Source: CAD feature listing. Evaluate the final solid. Frame: model axes, mm. A direction names the side the tool comes from. Give positions to 0.01 mm unless a question says otherwise; leave off trailing zeros. Loops run counter-clockwise (first coordinate to the right, second up) from the corner with the lowest first, then second, coordinate; pieces in that order, holes last. Notation, with made-up numbers: (-35.75, -3) - (-18.75, -3) arc R24 ccw to (-18.75, 22) - close; hole circle Ø10 at (79.25, 44.25). An arc over 180 degrees is marked (long way). Put each result on its own line as item: value.
```python
from build123d import *

# Parameters (mm, degrees)
BOSS_EXTRUDE1_DEPTH = 2.9972
FILLET1_R           = 1.27


with BuildPart() as part:
    # Sketch1 → Boss-Extrude1 (new body)
    with BuildSketch(Plane.XY):
        with BuildLine():
            Line((0, 0), (0, 15.24))
            Line((0, 15.24), (2.117246866, 15.24))
            ThreePointArc((2.117246866, 15.24), (6.0706, 8.001), (10.023953134, 15.24))
            Line((10.023953134, 15.24), (12.1412, 15.24))
            Line((12.1412, 15.24), (12.1412, 0))
            Line((12.1412, 0), (7.5692, 0))
            Line((7.5692, 0), (7.5692, 3.175))
            Line((7.5692, 3.175), (4.572, 3.175))
            Line((4.572, 3.175), (4.572, 0))
            Line((4.572, 0), (0, 0))
        make_face()
    extrude(amount=BOSS_EXTRUDE1_DEPTH)

    # Fillet1
    fillet1_edges = [part.edges().sort_by_distance(p)[0] for p in [
        (0, 0, 1.4986),
        (0, 15.24, 1.4986),
        (12.1412, 15.24, 1.4986),
        (12.1412, 0, 1.4986),
    ]]
    fillet(fillet1_edges, radius=FILLET1_R)


solid = part.part
```
1) Access query for faces 5 (the flat face through (4.572, 2, 1)), 6 (the cylindrical face through (0.362, 0.382, 1.52)). Directions: +Z, -Z, +X, -X, +Y, -Y. A direction counts if a zero-diameter tool reaches every point of the face in a straight line with its end or side. Return the directions, or none.
Check result:
face 5: +Z, -Z, -Y
face 6: +Z, -Z, -X, -Y
2) Mould query, pull axis X, two halves, no side actions, for faces 1 (the flat face through (9, 0, 1)), 2 (the cylindrical face through (6, 8, 1)), 3 (the flat face through (7.569, 2, 1)), 4 (the cylindrical face through (0.362, 14.858, 1.52)). Classes: pulls with the +X half, pulls with the -X half, needs draft (parallel to the pull), parting line crosses it, or undercut.
Check result:
face 1: needs draft
face 2: undercut
face 3: undercut
face 4: pulls with the -X half
3) Pin query (flat end, axial travel): P1, Ø0.9, axis at x = 6, z = 2, coming from the -Y side (3 decimals). Return the tip coordinate at first contact, or that it passes through.
Check result:
P1: y = 3.175
4) Section query A-A, the plane y = 12.7. Output: boundary loops of the cut face in (x, z), plus the area to 3 significant figures.
Check result:
outline: (0, 0) - (1.37, 0) - (1.37, 3) - (0, 3) - close; (10.77, 0) - (12.14, 0) - (12.14, 3) - (10.77, 3) - close
area: 8.22 mm²
5) Section query B-B, the plane z = 1.05. Output: boundary loops of the cut face in (x, y) (3 decimals), plus the area to 3 significant figures.
Check result:
outline: (0, 1.27) arc R1.27 ccw to (1.27, 0) - (4.572, 0) - (4.572, 3.175) - (7.569, 3.175) - (7.569, 0) - (10.871, 0) arc R1.27 ccw to (12.141, 1.27) - (12.141, 13.97) arc R1.27 ccw to (10.871, 15.24) - (10.024, 15.24) arc R4.699 cw (long way) to (2.117, 15.24) - (1.27, 15.24) arc R1.27 ccw to (0, 13.97) - close
area: 117 mm²
6) Material intervals for line 1 along X through (y, z) = (12.7, 2.1); line 2 along X through (y, z) = (3, 1.2); line 3 along Y through (x, z) = (7.25, 1.15) (3 decimals), sorted ascending. Write a range as [from, to].
Check result:
line 1: [0, 1.37], [10.77, 12.14]
line 2: [0, 4.57], [7.57, 12.14]
line 3: [3.175, 8.151]
7) Section query C-C, the plane y = 10.75. Output: boundary loops of the cut face in (x, z).
Check result:
outline: (0, 0) - (1.8, 0) - (1.8, 3) - (0, 3) - close; (10.35, 0) - (12.14, 0) - (12.14, 3) - (10.35, 3) - close
8) Section query D-D, the plane x = 6.75. Output: boundary loops of the cut face in (y, z) (3 decimals), plus the area to 3 significant figures.
Check result:
outline: (3.175, 0) - (8.05, 0) - (8.05, 2.997) - (3.175, 2.997) - close
area: 14.6 mm²
